Job drawing, mm, ordinate dimensions from the low corner. One solid piece. Coordinates: 2 decimals unless noted, no trailing zeros. Order: outer loops, then holes, each group sorted by start corner. A loop starts at its lowest first (then second) coordinate and runs counter-clockwise, first axis right, second up. Notation, with made-up numbers: (82, 10) - (89, 10) arc R23 cw to (89, 22) - close; hole circle Ø8 at (62, 75.5). An arc over 180 degrees is marked (long way). Return JSON: item names as keys, results as strings.
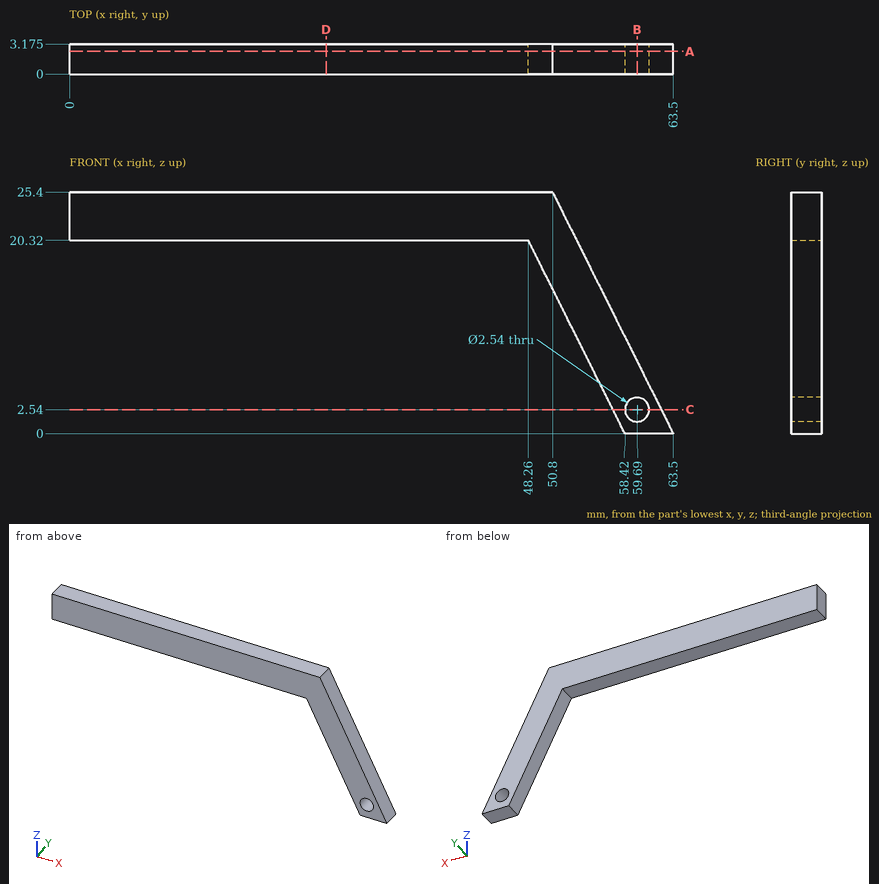
1. Probe L1, parallel to Z at x = 26, y = 1.5; L2, parallel to Z at x = 59.69, y = 1.7; L3, parallel to X at y = 0.8, z = 1.75 (3 decimals). List the from-to ranges inside material, lowest first.
Check values:
{"L1": "20.32 to 25.4", "L2": "0 to 1.27, 3.81 to 7.62", "L3": "57.545 to 58.696, 60.684 to 62.625"}
2. Cut at D-D on x = 27. Give the cut face in (y, z) (3 decimals), plus the area to 3 significant figures.
Check values:
{"outline": "(0, 20.32) - (3.175, 20.32) - (3.175, 25.4) - (0, 25.4) - close", "area": "16.1 mm²"}
3. Cut at A-A on y = 2.4. Give the cut face in (x, z), plus the area to 3 significant figures.
Check values:
{"outline": "(0, 20.32) - (48.26, 20.32) - (58.42, 0) - (63.5, 0) - (50.8, 25.4) - (0, 25.4) - close; hole circle Ø2.54 at (59.69, 2.54)", "area": "363 mm²"}
4. Drop flat-ended pins along their axis: pin 1 (1.5 mm diameter, centred on y = 2.5, z = 10.5, fed in from -X) (3 decimals); pin 2 (3 mm diameter, centred on x = 59.69, z = 2.54, fed in from +Y) (3 decimals); pin 3 (1.6 mm diameter, centred on x = 34, y = 2, fed in from -Z). Give the stop position or say it passes through.
Check values:
{"pin 1": "x = 52.795", "pin 2": "y = 3.175", "pin 3": "z = 20.32"}
5. Cut at C-C on z = 2.54. Give the cut face in (x, y) (3 decimals).
Check values:
{"outline": "(57.15, 0) - (58.42, 0) - (58.42, 3.175) - (57.15, 3.175) - close; (60.96, 0) - (62.23, 0) - (62.23, 3.175) - (60.96, 3.175) - close"}
6. Cut at B-B on x = 59.69. Give the cut face in (y, z) (3 decimals).
Check values:
{"outline": "(0, 0) - (3.175, 0) - (3.175, 1.27) - (0, 1.27) - close; (0, 3.81) - (3.175, 3.81) - (3.175, 7.62) - (0, 7.62) - close"}
